Part model, mm, in its own coordinate system. Face numbers are marked on the shaded views. A direction names the side the tool comes from. Give positions to 0.01 mm unless a question says otherwise; leave off trailing zeros. Order: outer loops, then holes, each group sorted by start corner. A loop starts at its lowest first (then second) coordinate and runs counter-clockwise, first axis right, second up. Notation, with made-up numbers: (-35, 85) - (-21, 85) arc R25 ccw to (-21, 115) - close; hole circle Ø10 at (23, 11.5). An arc over 180 degrees is marked (long way). One line per item, written item: value.
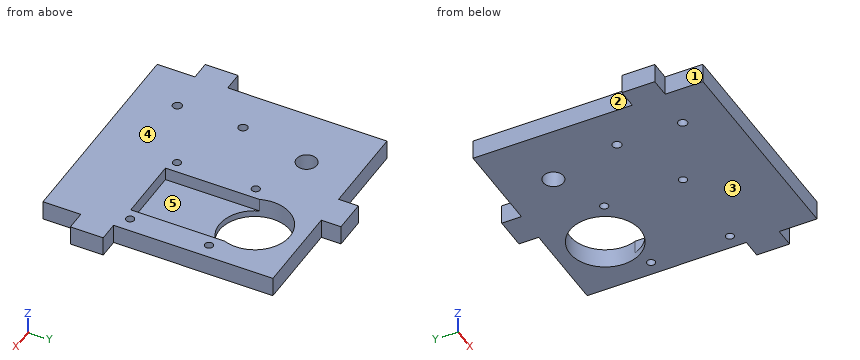
```python
from build123d import *

# Parameters (mm, degrees)
ESQUISSE1_W             = 66
ESQUISSE1_H             = 70
ESQUISSE1_R             = 10.75
ESQUISSE1_R_2           = 1.4
ESQUISSE1_R_3           = 3.1
BOSS_EXTRU_1_DEPTH      = 6
ESQUISSE2_W             = 10
ESQUISSE2_H             = 6
ESQUISSE2_W_2           = 6
ESQUISSE2_H_2           = 10
BOSS_EXTRU_3_DEPTH      = 6
ENL_V_MAT_EXTRU_3_DEPTH = 4
ESQUISSE4_R             = 1.25
ENL_V_MAT_EXTRU_4_DEPTH = 6


with BuildPart() as part:
    # Esquisse1 → Boss.-Extru.1 (new body)
    with BuildSketch(Plane.XY):
        with Locations((0, -20)):
            Rectangle(ESQUISSE1_W, ESQUISSE1_H)
        with Locations((15, 0)):
            Circle(ESQUISSE1_R, mode=Mode.SUBTRACT)
        with Locations((-20, -42)):
            Circle(ESQUISSE1_R_2, mode=Mode.SUBTRACT)
        with Locations((-20, -22)):
            Circle(ESQUISSE1_R_2, mode=Mode.SUBTRACT)
        with Locations((-15, 0)):
            Circle(ESQUISSE1_R_3, mode=Mode.SUBTRACT)
    extrude(amount=BOSS_EXTRU_1_DEPTH)

    # Esquisse2 → Boss.-Extru.3 (add)
    with BuildSketch(Plane.XY.offset(6)):
        with Locations((0, 18)):
            Rectangle(ESQUISSE2_W, ESQUISSE2_H)
        with Locations((-36, -38.5)):
            Rectangle(ESQUISSE2_W_2, ESQUISSE2_H_2)
        with Locations((36, -38.5)):
            Rectangle(ESQUISSE2_W_2, ESQUISSE2_H_2)
    extrude(amount=-BOSS_EXTRU_3_DEPTH)

    # Esquisse3 → Enlèv. mat.-Extru.3 (cut)
    with BuildSketch(Plane.XY.offset(6)):
        with BuildLine():
            Line((4.95, -3.815756806), (4.95, -32.465756806))
            Line((4.95, -32.465756806), (25.05, -32.465756806))
            Line((25.05, -32.465756806), (25.05, -3.815756806))
            ThreePointArc((25.05, -3.815756806), (15, -10.75), (4.95, -3.815756806))
        make_face()
    extrude(amount=-ENL_V_MAT_EXTRU_3_DEPTH, mode=Mode.SUBTRACT)

    # Esquisse4 → Enlèv. mat.-Extru.4 (cut)
    with BuildSketch(Plane.XY.offset(6)):
        with Locations((28.55, -6.815756806)):
            Circle(ESQUISSE4_R)
        with Locations((28.55, -30.815756806)):
            Circle(ESQUISSE4_R)
        with Locations((1.45, -30.815756806)):
            Circle(ESQUISSE4_R)
        with Locations((1.45, -6.815756806)):
            Circle(ESQUISSE4_R)
    extrude(amount=-ENL_V_MAT_EXTRU_4_DEPTH, mode=Mode.SUBTRACT)


solid = part.part
```
1) Slice it at B-B on y = -42. Write the cut outline in (x, z), then the cut area to 3 significant figures.
Answer:
outline: (-39, 0) - (-21.4, 0) - (-21.4, 6) - (-39, 6) - close; (-18.6, 0) - (39, 0) - (39, 6) - (-18.6, 6) - close
area: 451 mm2
2) Slice it at C-C on y = 0. Write the cut outline in (x, z), then the cut area to 3 significant figures.
Answer:
outline: (-33, 0) - (-18.1, 0) - (-18.1, 6) - (-33, 6) - close; (-11.9, 0) - (4.25, 0) - (4.25, 6) - (-11.9, 6) - close; (25.75, 0) - (33, 0) - (33, 6) - (25.75, 6) - close
area: 230 mm2
3) Wall check: line 1 along Y through (x, z) = (-20, 3.95); line 2 along Y through (x, z) = (28.55, 3.3); line 3 along X through (y, z) = (2, 5). Give the ranges that are in metal, low to high. Write a range as [from, to].
Answer:
line 1: y = [-55, -43.4], [-40.6, -23.4], [-20.6, 15]
line 2: y = [-55, -32.07], [-29.57, -8.07], [-5.57, 15]
line 3: x = [-33, -17.37], [-12.63, 4.44], [25.56, 33]
4) Slice it at A-A on x = 28.55. Write the cut outline in (y, z).
Answer:
outline: (-55, 0) - (-32.07, 0) - (-32.07, 6) - (-55, 6) - close; (-29.57, 0) - (-8.07, 0) - (-8.07, 6) - (-29.57, 6) - close; (-5.57, 0) - (15, 0) - (15, 6) - (-5.57, 6) - close
5) Which spindle directions (+Z, -Z, +X, -X, +Y, -Y) get a long thin tool onto all of the face, cutting with end or side? Do the marked faces 1, 2 and 3. Say none if no direction does.
Answer:
face 1: +Z, -Z, -X, -Y
face 2: +Z, -Z, -X, +Y
face 3: -Z, +X, -X, +Y, -Y
6) Drop flat-ended pins along their axis: P1, Ø2, axis at x = 28.55, y = -6.82, coming from the +Z side (3 decimals); P2, Ø2, axis at y = -21, z = 4, coming from the +X side; P3, Ø1.2, axis at x = 13.5, z = 4.5, coming from the +Y side; P4, Ø3, axis at y = 18, z = 2, coming from the -X side. Give the stop position or say it passes through.
Answer:
P1: passes through
P2: stops at x = 33
P3: stops at y = 15
P4: stops at x = -5
7) Slice it at D-D on z = 3.8. Count the separate pieces of the cut face and the enclosed holes in it, then the cut area to 3 significant figures.
Answer:
separate pieces: 1
enclosed holes: 8
area: 3,900 mm2
8) Two-plate mould, pull along Y, no slides. Class the marked faces 4 and 5: pulls with the +Y half, pulls with the -Y half, needs draft (parallel to the pull), parting line crosses it, or undercut.
Answer:
face 4: needs draft
face 5: undercut
